```python
from build123d import *

# Parameters (mm, degrees)
SKETCH1_W           = 90
SKETCH1_H           = 50
BOSS_EXTRUDE1_DEPTH = 40
SKETCH22_W          = 40
SKETCH22_H          = 13.4
CUT_EXTRUDE11_DEPTH = 9
SKETCH24_W          = 24
SKETCH24_H          = 13.4
CUT_EXTRUDE12_DEPTH = 31
SKETCH25_R          = 1.1
CUT_EXTRUDE13_DEPTH = 31
SKETCH31_W          = 25
SKETCH31_H          = 40
BOSS_EXTRUDE2_DEPTH = 50
SKETCH32_R          = 10
CUT_EXTRUDE15_DEPTH = 25
CHAMFER1_SIZE       = 10
CUT_EXTRUDE16_REACH = 142.357
SKETCH35_W          = 15
SKETCH35_H          = 20
SKETCH36_W          = 12
SKETCH36_H          = 12
SKETCH36_R          = 3.5
BOSS_EXTRUDE3_DEPTH = 10
SKETCH37_W          = 95.999091547
SKETCH37_H          = 21.11006165
CUT_EXTRUDE17_DEPTH = 100
SKETCH21_R          = 5
BOSS_EXTRUDE4_DEPTH = 15
SKETCH38_R          = 3.5
CUT_EXTRUDE18_DEPTH = 10
BOSS_EXTRUDE5_START = -7.186432503
SKETCH39_R          = 1.1
BOSS_EXTRUDE5_DEPTH = 7.186432503


with BuildPart() as part:
    # Sketch1 → Boss-Extrude1 (new body)
    with BuildSketch(Plane.XY):
        with Locations((-45, 25)):
            Rectangle(SKETCH1_W, SKETCH1_H)
    extrude(amount=BOSS_EXTRUDE1_DEPTH)

    # Sketch22 → Cut-Extrude11 (cut)
    with BuildSketch(Plane.XY.offset(40)):
        with Locations((-59.75, 25)):
            Rectangle(SKETCH22_W, SKETCH22_H)
    extrude(amount=-CUT_EXTRUDE11_DEPTH, mode=Mode.SUBTRACT)

    # Sketch24 → Cut-Extrude12 (cut)
    with BuildSketch(Plane.XY.offset(31)):
        with Locations((-59.75, 25)):
            Rectangle(SKETCH24_W, SKETCH24_H)
    extrude(amount=-CUT_EXTRUDE12_DEPTH, mode=Mode.SUBTRACT)

    # Sketch25 → Cut-Extrude13 (cut)
    with BuildSketch(Plane.XY.offset(31)):
        with Locations((-73.25, 25)):
            Circle(SKETCH25_R)
        with Locations((-46.25, 25)):
            Circle(SKETCH25_R)
    extrude(amount=-CUT_EXTRUDE13_DEPTH, mode=Mode.SUBTRACT)

    # Sketch31 → Boss-Extrude2 (add)
    with BuildSketch(Plane(origin=(0, 50, 0), x_dir=(1, 0, 0), z_dir=(0, 1, 0))):
        with Locations((-77.5, -20)):
            Rectangle(SKETCH31_W, SKETCH31_H)
    extrude(amount=BOSS_EXTRUDE2_DEPTH)

    # Sketch32 → Cut-Extrude15 (cut)
    with BuildSketch(Plane(origin=(-65, 0, 0), x_dir=(0, 0, -1), z_dir=(1, 0, 0))):
        with BuildLine():
            ThreePointArc((-40, 80), (-34.142135624, 94.142135624), (-20, 100))
            Line((-20, 100), (-40, 100))
            Line((-40, 100), (-40, 80))
        make_face()
        with BuildLine():
            ThreePointArc((-20, 100), (-5.857864376, 94.142135624), (0, 80))
            Line((0, 80), (0, 100))
            Line((0, 100), (-20, 100))
        make_face()
        with Locations((-20, 80)):
            Circle(SKETCH32_R)
    extrude(amount=-CUT_EXTRUDE15_DEPTH, mode=Mode.SUBTRACT)

    # Chamfer1
    chamfer1_edges = [part.edges().sort_by_distance(p)[0] for p in [
        (-65, 50, 20),
        (0, 50, 20),
        (0, 0, 20),
        (-90, 0, 20),
    ]]
    chamfer(chamfer1_edges, length=CHAMFER1_SIZE)

    # Cut-Extrude16: up to this face of the body (flat: up to its plane)
    cut_extrude16_end = Plane(part.part.faces().sort_by_distance((-47.75, 25, 15.5))[0])
    # Sketch35 → Cut-Extrude16 (cut, up to the picked face)
    with BuildSketch(Plane.ZY.offset(90), mode=Mode.PRIVATE) as cut_extrude16_sk1:
        with Locations((14.686432503, 25)):
            Rectangle(SKETCH35_W, SKETCH35_H)
    cut_extrude16_tool1 = split(extrude(cut_extrude16_sk1.sketch, amount=-CUT_EXTRUDE16_REACH, mode=Mode.PRIVATE), bisect_by=cut_extrude16_end, keep=Keep.BOTH, mode=Mode.PRIVATE)
    add(cut_extrude16_tool1.solids().sort_by(Axis((-90, 25, 14.686433), (1, 0, 0)))[0], mode=Mode.SUBTRACT)

    # Sketch36 → Boss-Extrude3 (add)
    # profile 1 of 2: a face of its own
    with BuildSketch(Plane.XY.offset(40)):
        with Locations((-65, -6)):
            Rectangle(SKETCH36_W, SKETCH36_H)
        with Locations((-65, -6)):
            Circle(SKETCH36_R, mode=Mode.SUBTRACT)
    # profile 2 of 2: a face of its own
    with BuildSketch(Plane.XY.offset(40)):
        with Locations((-25, -6)):
            Rectangle(SKETCH36_W, SKETCH36_H)
        with Locations((-25, -6)):
            Circle(SKETCH36_R, mode=Mode.SUBTRACT)
    extrude(amount=-BOSS_EXTRUDE3_DEPTH)

    # Sketch37 → Cut-Extrude17 (cut)
    with BuildSketch(Plane.XY.offset(40)):
        with Locations((-45.7868778, -3.784559742)):
            Rectangle(SKETCH37_W, SKETCH37_H)
    extrude(amount=-CUT_EXTRUDE17_DEPTH, mode=Mode.SUBTRACT)

    # Sketch21 → Boss-Extrude4 (add)
    with BuildSketch(Plane.XY.offset(40)):
        with Locations((-25, 25)):
            Circle(SKETCH21_R)
    extrude(amount=BOSS_EXTRUDE4_DEPTH)

    # Sketch38 → Cut-Extrude18 (cut)
    with BuildSketch(Plane.XY.offset(55)):
        with Locations((-25, 25)):
            Circle(SKETCH38_R)
    extrude(amount=-CUT_EXTRUDE18_DEPTH, mode=Mode.SUBTRACT)

    # Sketch39 → Boss-Extrude5 (add)
    with BuildSketch(Plane(origin=(0, 0, 0), x_dir=(-1, 0, 0), z_dir=(0, 0, -1)).offset(BOSS_EXTRUDE5_START)):
        with Locations(Location((46.25, 25, 0), (0, 0, 180))):
            Circle(SKETCH39_R)
        with Locations(Location((73.25, 25, 0), (0, 0, 180))):
            Circle(SKETCH39_R)
    extrude(amount=BOSS_EXTRUDE5_DEPTH)


solid = part.part
```
Geometry check sheet. Reference: the model listing, model coordinates, mm. A direction names the side the tool comes from. Give positions to 0.01 mm unless a question says otherwise; leave off trailing zeros. Write each loop counter-clockwise with the first axis right and the second up, starting at its lowest first coordinate (ties: lowest second). Pieces come first, ordered by that corner, then holes.
1) Gauge pin test, flat ends, axial feed: pin 1 (14.5 mm diameter, centred on x = -50, z = 29.5, fed in from +Y); pin 2 (6 mm diameter, centred on x = -39.5, z = 36.5, fed in from +Y); pin 3 (2.5 mm diameter, centred on x = -75.5, y = 27, fed in from +Z). Record the tip position at first contact, or that the pin passes through.
2) Section check C-C, the plane z = 24. Record the boundary of the cut face in (x, y), and give its area (3 significant figures).
3) Section check D-D, the plane x = -76.5. Record the boundary of the cut face in (y, z).
4) Material ranges on L1, parallel to Y at x = -73.5, z = 20; L2, parallel to X at y = 25, z = 12; L3, parallel to X at y = 20.5, z = 10, recorded low to high.
5) Release check for a two-part mould opening along Z. For faces 1 (the flat face through (-46, 25, 7.186)), 2 (the flat face through (-71.75, 25, 4)), 3 (the flat face through (-74, 25, 7.186)) record: pulls with the +Z half, pulls with the -Z half, needs draft (parallel to the pull), parting line crosses it, or undercut.
6) Section check B-B, the plane x = -49. Record the boundary of the cut face in (y, z), and give its area (3 significant figures).
7) Access from +Z, -Z, +X, -X, +Y, -Y to the whole of each face (thin tool, end or side, straight path). Record for faces 4 (the flat face through (-69, 35, 15)), 5 (the flat face through (-39.75, 25, 36)), 6 (the flat face through (-47.75, 25, 16)), 7 (the flat face through (-60, 18.3, 4)).
8) Section check A-A, the plane z = 18. Record the boundary of the cut face in (x, y), and give its area (3 significant figures).
Computed:
1. pin 1: stops at y = 52.25
1. pin 2: stops at y = 50
1. pin 3: stops at z = 31
2. outline: (-90, 10) - (-86.77, 6.77) - (-3.23, 6.77) - (0, 10) - (0, 40) - (-10, 50) - (-55, 50) - (-65, 60) - (-65, 70.83) - (-90, 70.83) - close; (-90, 89.17) - (-65, 89.17) - (-65, 99.6) - (-90, 99.6) - close; hole circle Ø2.2 at (-73.25, 25); hole (-71.75, 18.3) - (-47.75, 18.3) - (-47.75, 31.7) - (-71.75, 31.7) - close; hole circle Ø2.2 at (-46.25, 25)
2. area: 4,330 mm2
3. outline: (6.77, 0) - (80, 0) arc R20 ccw to (80, 40) - (31.7, 40) - (31.7, 31) - (18.3, 31) - (18.3, 40) - (6.77, 40) - close; hole (15, 7.19) - (35, 7.19) - (35, 22.19) - (15, 22.19) - close; hole circle Ø20 at (80, 20)
4. L1: y = 6.77 to 15, 35 to 70, 90 to 100
4. L2: x = -47.75 to -47.35, -45.15 to 0
4. L3: x = -47.75 to 0
5. face 1: pulls with the +Z half
5. face 2: needs draft
5. face 3: undercut
6. outline: (6.77, 0) - (18.3, 0) - (18.3, 7.19) - (15, 7.19) - (15, 22.19) - (18.3, 22.19) - (18.3, 40) - (6.77, 40) - close; (31.7, 0) - (50, 0) - (50, 40) - (31.7, 40) - (31.7, 22.19) - (35, 22.19) - (35, 7.19) - (31.7, 7.19) - close
6. area: 1,090 mm2
7. face 4: -X
7. face 5: +Z
7. face 6: none
7. face 7: +Z, -Z
8. outline: (-90, 10) - (-86.77, 6.77) - (-3.23, 6.77) - (0, 10) - (0, 40) - (-10, 50) - (-55, 50) - (-65, 60) - (-65, 70.2) - (-90, 70.2) - (-90, 35) - (-47.75, 35) - (-47.75, 15) - (-90, 15) - close; (-90, 89.8) - (-65, 89.8) - (-65, 99.9) - (-90, 99.9) - close; hole circle Ø2.2 at (-46.25, 25)
8. area: 3,790 mm2
